For this review, take the finished solid that the model builds, in its own axes (mm). A direction names the side the tool comes from. Give positions to 0.01 mm unless a question says otherwise; leave off trailing zeros. Write each loop counter-clockwise with the first axis right and the second up, starting at its lowest first coordinate (ties: lowest second). Pieces come first, ordered by that corner, then holes.
1) For P1, Ø6, axis at x = -10, z = 35.5, coming from the +Y side; P2, Ø1, axis at x = 12, y = -1.5, coming from the -Z side; P3, Ø5, axis at x = 17.5, y = 0, coming from the +Z side; P4, Ø1.6, axis at x = -12, y = -3, coming from the +Z side, all flat-tipped, find the tip position at first contact; note any pin that passes through.
2) We need section B-B on y = 15. Give the boundary of the cut face in (x, z).
3) We need section A-A on x = -17.5. Give the boundary of the cut face in (y, z), and give its area (3 significant figures).
4) Draft analysis for pull direction Y (two halves, no side actions). For faces 1 (the face through (0, 17.5, 1)), 2 (the face through (-16.18, 16.08, 0.99)), 3 (the face through (8.8, -11.49, 35.21)), state which applies: pulls with the +Y half, pulls with the -Y half, needs draft (parallel to the pull), parting line crosses it, or undercut.
5) We need section D-D on z = 25.5. Give the boundary of the cut face in (x, y).
6) We need section C-C on y = 6. Give the boundary of the cut face in (x, z), and give its area (3 significant figures).
7) Machinability: for faces 4 (the face through (-12, -3, 10)), 5 (the face through (5, -11, 64)), 6 (the face through (6.056, 6.165, 0.986)), which of the approach directions +Z, -Z, +X, -X, +Y, -Y give a long, thin tool a straight path to every point of the face, cutting with its end or side? Answer none if there is none.
8) Wall thickness on line 1 along Y through (x, z) = (15, 1.25); line 2 along Y through (x, z) = (8, 1); line 3 along Z through (x, y) = (-13, 7.5): over which ranges is each line inside the solid? List them lowest first.
from build123d import *

# Parameters (mm, degrees)
F1_W     = 21
F1_H     = 21
F1_R     = 1.1
F1_H_2   = 2
F1_W_2   = 10
F1_H_3   = 15
F1_R_2   = 1.6
F2_DEPTH = 2
F3_DEPTH = 90
F4_DEPTH = 10
F5_SIZE  = 7.99999
F7_DEPTH = 25


# Not quite as in the source:
# - a fillet or chamfer is up to 0.001 mm smaller than in the source, because OpenCascade refuses the exact size


with BuildPart() as f2:
    # F1 (on Top) → F2 (new body)
    with BuildSketch(Plane.XY):
        Rectangle(F1_W, F1_H)
        with Locations((-8, -8)):
            Circle(F1_R, mode=Mode.SUBTRACT)
        with Locations((8, -8)):
            Circle(F1_R, mode=Mode.SUBTRACT)
        with Locations((-8, 8)):
            Circle(F1_R, mode=Mode.SUBTRACT)
        Polygon((-10, 2.2218254069), (-2.2218254069, 10), (2.2218254069, 10), (10, 2.2218254069), (10, -2.2218254069), (2.2218254069, -10), (-2.2218254069, -10), (-10, -2.2218254069), align=None, mode=Mode.SUBTRACT)
        with Locations((8, 8)):
            Circle(F1_R, mode=Mode.SUBTRACT)
        Polygon((-10.5, 12.5), (-12.5, 12.5), (-12.5, 7.8503944539), (-12.5, -7.1496055461), (-12.5, -10.5), (-10.5, -10.5), (-10.5, 10.5), align=None)
        with Locations((0, 11.5)):
            Rectangle(F1_W, F1_H_2)
        Polygon((12.5, 12.5), (10.5, 12.5), (10.5, 10.5), (10.5, -10.5), (12.5, -10.5), (12.5, -7.1496055461), (12.5, 7.8503944539), align=None)
        with Locations((-17.5, 0.3503944539)):
            Rectangle(F1_W_2, F1_H_3)
        with Locations((-17.5, 0)):
            Circle(F1_R_2, mode=Mode.SUBTRACT)
        with Locations((17.5, 0.3503944539)):
            Rectangle(F1_W_2, F1_H_3)
        with Locations((17.5, 0)):
            Circle(F1_R_2, mode=Mode.SUBTRACT)
        Polygon((-12.5, 7.8503944539), (-12.5, 12.5), (-10.5, 12.5), (10.5, 12.5), (12.5, 12.5), (12.5, 7.8503944539), (22.5, 7.8503944539), (22.5, 17.5), (-22.5, 17.5), (-22.5, 7.8503944539), align=None)
        with Locations((-15, 15)):
            Circle(F1_R_2, mode=Mode.SUBTRACT)
        with Locations((15, 15)):
            Circle(F1_R_2, mode=Mode.SUBTRACT)
        Polygon((-12.5, -10.5), (-12.5, -7.1496055461), (-22.5, -7.1496055461), (-22.5, -17.5), (22.5, -17.5), (22.5, -7.1496055461), (12.5, -7.1496055461), (12.5, -10.5), (12.5, -12.5), (-12.5, -12.5), align=None)
        with Locations((-15, -15)):
            Circle(F1_R_2, mode=Mode.SUBTRACT)
        with Locations((15, -15)):
            Circle(F1_R_2, mode=Mode.SUBTRACT)
        Polygon((10.5, -10.5), (-10.5, -10.5), (-12.5, -10.5), (-12.5, -12.5), (12.5, -12.5), (12.5, -10.5), align=None)
    extrude(amount=F2_DEPTH)

    # F1 (on Top) → F3 (join)
    with BuildSketch(Plane.XY):
        Polygon((10.5, -10.5), (-10.5, -10.5), (-12.5, -10.5), (-12.5, -12.5), (12.5, -12.5), (12.5, -10.5), align=None)
    extrude(amount=F3_DEPTH)

    # F1 (on Top) → F4 (join)
    with BuildSketch(Plane.XY):
        Polygon((12.5, 12.5), (10.5, 12.5), (10.5, 10.5), (10.5, -10.5), (12.5, -10.5), (12.5, -7.1496055461), (12.5, 7.8503944539), align=None)
        Polygon((-10.5, 12.5), (-12.5, 12.5), (-12.5, 7.8503944539), (-12.5, -7.1496055461), (-12.5, -10.5), (-10.5, -10.5), (-10.5, 10.5), align=None)
        Polygon((10.5, -10.5), (-10.5, -10.5), (-12.5, -10.5), (-12.5, -12.5), (12.5, -12.5), (12.5, -10.5), align=None)
    extrude(amount=F4_DEPTH)

    # F5 (size 8 in the source; OpenCascade refuses exactly that, so slightly less here)
    f5_edges = [f2.edges().sort_by_distance(p)[0] for p in [
        (11.5, 12.5, 10),
        (-11.5, 12.5, 10),
    ]]
    chamfer(f5_edges, length=F5_SIZE)

    # F6 (on face) → F7 (cut)
    with BuildSketch(Plane(origin=(0, -10.5, 0), x_dir=(-1, 0, 0), z_dir=(0, 1, 0))):
        Polygon((-12.5, 90), (-12.5, 31.766526401), (-5, 38.7480794755), (-5, 90), align=None)
        Polygon((5, 38.7480794755), (12.5, 31.766526401), (12.5, 90), (5, 90), align=None)
    extrude(amount=-F7_DEPTH, mode=Mode.SUBTRACT)


solid = f2.part
Results list:
1. P1: stops at y = -10.5
1. P2: stops at z = 0
1. P3: stops at z = 2
1. P4: stops at z = 10
2. outline: (-22.5, 0) - (-16.6, 0) - (-16.6, 2) - (-22.5, 2) - close; (-13.4, 0) - (13.4, 0) - (13.4, 2) - (-13.4, 2) - close; (16.6, 0) - (22.5, 0) - (22.5, 2) - (16.6, 2) - close
3. outline: (-17.5, 0) - (-1.6, 0) - (-1.6, 2) - (-17.5, 2) - close; (1.6, 0) - (17.5, 0) - (17.5, 2) - (1.6, 2) - close
3. area: 63.6 mm2
4. face 1: pulls with the +Y half
4. face 2: undercut
4. face 3: needs draft
5. outline: (-12.5, -12.5) - (12.5, -12.5) - (12.5, -10.5) - (-12.5, -10.5) - close
6. outline: (-22.5, 0) - (-6.22, 0) - (-6.22, 2) - (-10.5, 2) - (-10.5, 8.5) - (-12.5, 8.5) - (-12.5, 2) - (-22.5, 2) - close; (6.22, 0) - (22.5, 0) - (22.5, 2) - (12.5, 2) - (12.5, 8.5) - (10.5, 8.5) - (10.5, 2) - (6.22, 2) - close
6. area: 91.1 mm2
7. face 4: +Z, +X, -X, +Y
7. face 5: +Z, +X, +Y, -Y
7. face 6: +Z, -Z
8. line 1: y = -17.5 to -16.6, -13.4 to 13.4, 16.6 to 17.5
8. line 2: y = -17.5 to -9.1, -6.9 to -4.22, 4.22 to 6.9, 9.1 to 17.5
8. line 3: z = 0 to 2
